```python
from build123d import *

# Parameters (mm, degrees)
F0_R     = 2.5
F1_DEPTH = 8
F2_R     = 0.5
F4_R     = 1
F5_DEPTH = 16.0046179008


with BuildPart() as f1:
    # F0 (on Front) → F1 (new body)
    with BuildSketch(Plane.XZ):
        with BuildLine():
            ThreePointArc((-3.7562448003, -7.625), (-2.2912878475, -5.7212807378), (0, -5))
            Line((0, -5), (2.9270166538, -5))
            ThreePointArc((2.9270166538, -5), (6.089294314, -3.4494897428), (6.8, 0))
            Line((6.8, 0), (6.8, 4.1654431261))
            ThreePointArc((6.8, 4.1654431261), (7.6768943744, 6.9938702509), (10, 8.830204642))
            Line((10, 8.830204642), (10, 12.5))
            Line((10, 12.5), (3.7225915585, 12.5))
            ThreePointArc((3.7225915585, 12.5), (1.2642823664, 11.3254788413), (-1.3759608742, 11.9977136707))
            ThreePointArc((-1.3759608742, 11.9977136707), (-3.8097222151, 6.2411904989), (-4.1388034343, 0))
            ThreePointArc((-4.1388034343, 0), (-3.9545717948, -3.3296918319), (-6.3576388045, -5.6418462255))
            ThreePointArc((-6.3576388045, -5.6418462255), (-5.1532402541, -6.7597422202), (-3.7562448003, -7.625))
        make_face()
        Circle(F0_R, mode=Mode.SUBTRACT)
    extrude(amount=F1_DEPTH)

    # F2
    f2_edges = [f1.edges().sort_by_distance(p)[0] for p in [
        (10, -4, 12.5),
        (-1.375961, -4, 11.997714),
        (-6.357639, -4, -5.641846),
        (-3.756245, -4, -7.625),
        (10, -4, 8.830205),
    ]]
    fillet(f2_edges, radius=F2_R)

    # F4 (on face) → F5 (cut, through all)
    with BuildSketch(Plane.YZ.offset(10)):
        with Locations((-4, 0)):
            Circle(F4_R)
    extrude(amount=-F5_DEPTH, mode=Mode.SUBTRACT)


solid = f1.part
```
Build history of the part. All positions in model axes, mm. A direction names the side the tool comes from. Round coordinates to 2 decimals unless told otherwise and drop trailing zeros. Write each loop counter-clockwise with the first axis right and the second up, starting at its lowest first coordinate (ties: lowest second). Pieces come first, ordered by that corner, then holes.
1) Drill centre lines: probe 1 along X at (y, z) = (-2.5, 1); probe 2 along X at (y, z) = (-2.5, 0); probe 3 along X at (y, z) = (-7.5, 8.25). Where is each one in solid material? Low to high.
2) Band-saw the part on A-A, the plane x = 0.25. List the corners of the cut face in (y, z).
3) Band-saw the part on B-B, the plane z = 2.25. List the corners of the cut face in (x, y), and give its area (3 significant figures).
4) Mould opens along Z. For faces 1 (the flat face through (1, -4, -5)), 2 (the flat face through (7, -4, 12.5)), 3 (the cylindrical face through (-3.833, -3.944, -2.971)) say: +Z half, -Z half, draft (parallel to the pull), parting line (faces both ways), or undercut.
5) Pin check, flat tips, straight feed: pin 1 (2 mm diameter, centred on y = -1.5, z = 0, fed in from +X); pin 2 (2.5 mm diameter, centred on y = -4, z = 0, fed in from -X); pin 3 (0.9 mm diameter, centred on x = 1, y = -3.5, fed in from -Z); pin 4 (4 mm diameter, centred on x = 0, z = 0, fed in from +Y). Stop position of each tip, or through.
6) Band-saw the part on D-D, the plane x = 4.25. List the corners of the cut face in (y, z).
7) 3-axis set-ups, long thin cutter, end or side, ignore diameter. For faces 4 (the cylindrical face through (1.15, -3.94, -2.22)), 5 (the flat face through (6.8, -4, 2)): which of +Z, -Z, +X, -X, +Y, -Y reach the whole face in a straight line?
8) Band-saw the part on C-C, the plane z = -0.25. List the corners of the cut face in (x, y).
Ans:
1. probe 1: x = -4.23 to -2.29, 2.29 to 6.8
1. probe 2: x = -4.14 to -2.5, 2.5 to 6.8
1. probe 3: x = -3.22 to 8.92
2. outline: (-8, -5) - (0, -5) - (0, -2.49) - (-8, -2.49) - close; (-8, 2.49) - (0, 2.49) - (0, 11.35) - (-8, 11.35) - close
3. outline: (-4.27, -8) - (-1.09, -8) - (-1.09, 0) - (-4.27, 0) - close; (1.09, -8) - (6.8, -8) - (6.8, 0) - (1.09, 0) - close
3. area: 71.1 mm2
4. face 1: -Z half
4. face 2: +Z half
4. face 3: undercut
5. pin 1: stops at x = 6.93
5. pin 2: stops at x = -4.25
5. pin 3: stops at z = -5
5. pin 4: passes through
6. outline: (-8, -4.77) - (0, -4.77) - (0, 12.5) - (-8, 12.5) - close; hole circle Ø2 at (-4, 0)
7. face 4: +Y, -Y
7. face 5: +X, +Y, -Y
8. outline: (-4.02, -8) - (-2.49, -8) - (-2.49, -4.97) - (-4.02, -4.97) - close; (-4.02, -3.03) - (-2.49, -3.03) - (-2.49, 0) - (-4.02, 0) - close; (2.49, -8) - (6.86, -8) - (6.86, -4.97) - (2.49, -4.97) - close; (2.49, -3.03) - (6.86, -3.03) - (6.86, 0) - (2.49, 0) - close
